```python
from build123d import *

# Parameters (mm, degrees)
SKETCH1_R               = 2.6
BOSS_EXTRUDE1_DEPTH     = 35
CUT_EXTRUDE3_DEPTH      = 10
CUT_EXTRUDE4_DEPTH      = 67.997971518
CUT_EXTRUDE4_DEPTH_BACK = 67.997971518
SKETCH5_R               = 1
CUT_EXTRUDE5_DEPTH      = 44.084608481
FILLET1_R               = 3
CUT_EXTRUDE6_DEPTH      = 67.997971643
CUT_EXTRUDE6_DEPTH_BACK = 67.997971643
FILLET2_R               = 1


with BuildPart() as part:
    # Sketch1 → Boss-Extrude1 (new body)
    with BuildSketch(Plane.XY):
        with BuildLine():
            Line((-19.191312838, -37.02606043), (-15.551610496, -47.02606043))
            ThreePointArc((-15.551610496, -47.02606043), (-14.453261942, -48.457456133), (-12.732532633, -49))
            Line((-12.732532633, -49), (12.732532633, -49))
            ThreePointArc((12.732532633, -49), (14.453261942, -48.457456133), (15.551610496, -47.02606043))
            Line((15.551610496, -47.02606043), (19.191312838, -37.02606043))
            ThreePointArc((19.191312838, -37.02606043), (18.829691109, -34.279270691), (16.372234976, -33))
            Line((16.372234976, -33), (12.115523886, -33))
            ThreePointArc((12.115523886, -33), (10.394794577, -33.542543867), (9.296446024, -34.97393957))
            Line((9.296446024, -34.97393957), (7.093654177, -41.02606043))
            ThreePointArc((7.093654177, -41.02606043), (5.995305623, -42.457456133), (4.274576314, -43))
            Line((4.274576314, -43), (-4.274576314, -43))
            ThreePointArc((-4.274576314, -43), (-5.995305623, -42.457456133), (-7.093654177, -41.02606043))
            Line((-7.093654177, -41.02606043), (-9.296446024, -34.97393957))
            ThreePointArc((-9.296446024, -34.97393957), (-10.394794577, -33.542543867), (-12.115523886, -33))
            Line((-12.115523886, -33), (-16.372234976, -33))
            ThreePointArc((-16.372234976, -33), (-18.829691109, -34.279270691), (-19.191312838, -37.02606043))
        make_face()
        with Locations(Location((-14.944086969, -37, 0), (0, 0, 180))):
            Circle(SKETCH1_R, mode=Mode.SUBTRACT)
        with Locations(Location((14.944086969, -37, 0), (0, 0, 180))):
            Circle(SKETCH1_R, mode=Mode.SUBTRACT)
    extrude(amount=BOSS_EXTRUDE1_DEPTH)

    # Sketch4 → Cut-Extrude3 (cut, symmetric)
    with BuildSketch(Plane(origin=(0, 0, 0), x_dir=(0, 0, -1), z_dir=(1, 0, 0))):
        Polygon((-35, -49), (-11, -49), (-3.53907747, -33), (-35, -33), align=None)
    extrude(amount=CUT_EXTRUDE3_DEPTH, both=True, mode=Mode.SUBTRACT)

    # Sketch5 → Cut-Extrude4 (cut, two sides: drawn at the far end of the back side and taken through both)
    with BuildSketch(Plane.ZY.offset(-10).offset(-CUT_EXTRUDE4_DEPTH_BACK)):
        with Locations((21, -45.3)):
            Circle(SKETCH5_R)
    extrude(amount=CUT_EXTRUDE4_DEPTH + CUT_EXTRUDE4_DEPTH_BACK, mode=Mode.SUBTRACT)

    # Sketch6 → Cut-Extrude5 (cut, through all)
    with BuildSketch(Plane.XZ.offset(49)):
        Polygon((-11.532532633, 0), (11.532532633, 0), (8.645781287, 5), (-8.645781287, 5), align=None)
    extrude(amount=-CUT_EXTRUDE5_DEPTH, mode=Mode.SUBTRACT)

    # Fillet1
    fillet1_edges = [part.edges().sort_by_distance(p)[0] for p in [
        (-8.645781287, -42.88081312, 5),
        (8.645781287, -42.88081312, 5),
    ]]
    fillet(fillet1_edges, radius=FILLET1_R)

    # Sketch7 → Cut-Extrude6 (cut, two sides: drawn at the far end of the back side and taken through both)
    with BuildSketch(Plane.ZY.offset(-10).offset(-CUT_EXTRUDE6_DEPTH_BACK)):
        with BuildLine():
            Line((35, -42), (35, -49))
            Line((35, -49), (10, -49))
            ThreePointArc((10, -49), (22.980754986, -47.216982092), (35, -42))
        make_face()
    extrude(amount=CUT_EXTRUDE6_DEPTH + CUT_EXTRUDE6_DEPTH_BACK, mode=Mode.SUBTRACT)

    # Fillet2
    fillet2_edges = [part.edges().sort_by_distance(p)[0] for p in [
        (-10, -41.431305772, 7.470659919),
        (10, -41.431305772, 7.470659919),
    ]]
    fillet(fillet2_edges, radius=FILLET2_R)


solid = part.part
```
The model under review builds one solid part; all positions refer to its coordinate system, in mm. A direction names the side the tool comes from. Give positions to 0.01 mm unless a question says otherwise; leave off trailing zeros. Write each loop counter-clockwise with the first axis right and the second up, starting at its lowest first coordinate (ties: lowest second). Pieces come first, ordered by that corner, then holes.
(1) Consider section C-C, the plane x = 14.5. Give the boundary of the cut face in (y, z), and give its area (3 significant figures).
(2) For P1, Ø2.5, axis at y = -45.3, z = 21, coming from the -X side; P2, Ø1.6, axis at y = -45.3, z = 21, coming from the -X side; P3, Ø3, axis at x = 15, z = 17.5, coming from the -Y side; P4, Ø6, axis at y = -35.5, z = 13.5, coming from the +X side, all flat-tipped, find the tip position at first contact; note any pin that passes through.
(3) Consider section A-A, the plane z = 29. Give the boundary of the cut face in (x, y).
(4) The part is to be moulded in two halves that separate along X. For faces 6 (the flat face through (14, -33, 17)), 7 (the cylindrical face through (-18.81, -34.25, 17.26)), 8 (the cylindrical face through (-14.38, -34.46, 17.26)), 9 (the flat face through (10, -40, 20)), say which applies: released by +X, released by -X, zero draft, split by the parting line, or undercut.
(5) To check wall thickness, follow L1, parallel to X at y = -37, z = 15; L2, parallel to X at y = -36.5, z = 30; L3, parallel to Y at x = -15, z = 21. State the ranges of each line that lie inside material, in increasing order.
(6) Consider section D-D, the plane y = -45.75. Give the number of separate pieces and of enclosed holes in the cut face, and give its area (3 significant figures).
(7) Tool access review of faces 1 (the flat face through (0, -49, 7)), 2 (the flat face through (-15, -41, 0)), 3 (the cylindrical face through (11.141, -33.163, 17.255)), 4 (the flat face through (-10.51, -41.14, 1.77)), 5 (the cylindrical face through (-9.7, -41.57, 7.85)): name each direction out of +Z, -Z, +X, -X, +Y, -Y from which nothing blocks a thin tool from reaching the whole face with its end or side.
(8) Consider section B-B, the plane z = 21. Give the boundary of the cut face in (x, y), and give its area (3 significant figures).
Returned:
1. outline: (-48.42, 0) - (-39.56, 0) - (-39.56, 35) - (-42, 35) arc R48.14 ccw to (-48.42, 17.42) - close; (-34.44, 0) - (-33, 0) - (-33, 35) - (-34.44, 35) - close; hole circle Ø2 at (-45.3, 21)
1. area: 312 mm2
2. P1: stops at x = -16.63
2. P2: passes through
2. P3: stops at y = -48.6
2. P4: stops at x = 19.37
3. outline: (-19.19, -37.03) - (-16.26, -45.09) - (-10, -45.09) - (-10, -33.87) arc R3 ccw to (-12.12, -33) - (-16.37, -33) arc R3 ccw to start; (10, -45.09) - (16.26, -45.09) - (19.19, -37.03) arc R3 ccw to (16.37, -33) - (12.12, -33) arc R3 ccw to (10, -33.87) - close; hole circle Ø5.2 at (-14.94, -37); hole circle Ø5.2 at (14.94, -37)
4. face 6: zero draft
4. face 7: released by -X
4. face 8: undercut
4. face 9: undercut
5. L1: x = -19.2 to -17.54, -12.34 to -10, 10 to 12.34, 17.54 to 19.2
5. L2: x = -19.33 to -17.5, -12.39 to -10, 10 to 12.39, 17.5 to 19.33
5. L3: y = -47.73 to -46.3, -44.3 to -39.6, -34.4 to -33
6. separate pieces: 3
6. enclosed holes: 0
6. area: 398 mm2
7. face 1: +Z, -Z, +X, -X, -Y
7. face 2: -Z, +X, -X, +Y, -Y
7. face 3: +Z, -Z, +Y
7. face 4: -Z, +Y, -Y
7. face 5: +Z, +Y
8. outline: (-19.19, -37.03) - (-16.54, -44.3) - (-10, -44.3) - (-10, -33.87) arc R3 ccw to (-12.12, -33) - (-16.37, -33) arc R3 ccw to start; (-15.82, -46.3) - (-15.55, -47.03) arc R3 ccw to (-15.19, -47.73) - (-10, -47.73) - (-10, -46.3) - close; (10, -47.73) - (15.19, -47.73) arc R3 ccw to (15.55, -47.03) - (15.82, -46.3) - (10, -46.3) - close; (10, -44.3) - (16.54, -44.3) - (19.19, -37.03) arc R3 ccw to (16.37, -33) - (12.12, -33) arc R3 ccw to (10, -33.87) - close; hole circle Ø5.2 at (-14.94, -37); hole circle Ø5.2 at (14.94, -37)
8. area: 158 mm2
